Check sheet for the modelled part. Datum: model origin and axes. Units: mm. Round coordinates to 2 decimals unless told otherwise and drop trailing zeros. Write each loop counter-clockwise with the first axis right and the second up, starting at its lowest first coordinate (ties: lowest second). Pieces come first, ordered by that corner, then holes. Notation, with made-up numbers: (-35.75, 26) -> (8.25, 26) arc R23 cw to (8.25, 52) -> close; hole circle Ø3 at (28, -38). An arc over 180 degrees is marked (long way). Put each result on its own line as item: value. Start each with the question number.
from build123d import *

# Parameters (mm, degrees)
SALIENTE_EXTRUIR1_DEPTH = 3


with BuildPart() as part:
    # Model → Saliente-Extruir1 (new body)
    with BuildSketch(Plane.XY):
        with BuildLine():
            Line((49.555981249, 5.697120887), (50.217934692, 7.253298598))
            Line((50.217934692, 7.253298598), (50.092452983, 8.243189758))
            ThreePointArc((50.092452983, 8.243189758), (27.621595202, 14.792954102), (10.694790748, 30.958415843))
            Line((10.694790748, 30.958415843), (9.611017038, 30.557274304))
            Line((9.611017038, 30.557274304), (8.582065308, 29.179502343))
            ThreePointArc((8.582065308, 29.179502343), (9.359106699, 24.192582613), (11.075472958, 19.446294739))
            ThreePointArc((11.075472958, 19.446294739), (24.748133849, 6.443892033), (43.61000442, 5.960187025))
            ThreePointArc((43.61000442, 5.960187025), (46.607144549, 6.374545334), (49.555981249, 5.697120887))
        make_face()
    extrude(amount=SALIENTE_EXTRUIR1_DEPTH)


solid = part.part
1. Gauge pin test, flat end, axial feed: P1, Ø1, axis at x = 41.5, z = 2.5, coming from the +Y side. Record the tip position at first contact, or that the pin passes through.
2. Section check C-C, the plane x = 28. Enter the section's corners in (y, z).
3. Section check B-B, the plane y = 11.5. Enter the section's corners in (x, z), then the cut area to 3 significant figures.
4. Material ranges on L1, parallel to X at y = 18.75, z = 2.1; L2, parallel to Y at x = 25.5, z = 2.7; L3, parallel to Y at x = 13, z = 1.4, recorded low to high. Write a range as [from, to].
5. Section check A-A, the plane z = 2.4. Enter the section's corners in (x, y), then the cut area to 3 significant figures.
6. Draft check along X on faces 1 (the flat face through (10.16, 30.76, 1.48)), 2 (the cylindrical face through (46.565, 6.376, 1.479)), 3 (the flat face through (25, 13, 3)), 4 (the flat face through (49.88, 6.46, 1.48)). Enter one of: released by +X, released by -X, zero draft, split by the parting line, or undercut.
Reply:
1. P1: stops at y = 9.5
2. outline: (5.34, 0) -> (14.58, 0) -> (14.58, 3) -> (5.34, 3) -> close
3. outline: (16.89, 0) -> (34.52, 0) -> (34.52, 3) -> (16.89, 3) -> close
3. area: 52.9 mm2
4. L1: x = [11.42, 21.77]
4. L2: y = [6.15, 16.09]
4. L3: y = [16.06, 27.66]
5. outline: (8.58, 29.18) arc R26.27 ccw to (43.61, 5.96) arc R8.38 cw to (49.56, 5.7) -> (50.22, 7.25) -> (50.09, 8.24) arc R49.36 cw to (10.69, 30.96) -> (9.61, 30.56) -> close
5. area: 319 mm2
6. face 1: released by -X
6. face 2: undercut
6. face 3: zero draft
6. face 4: released by +X
